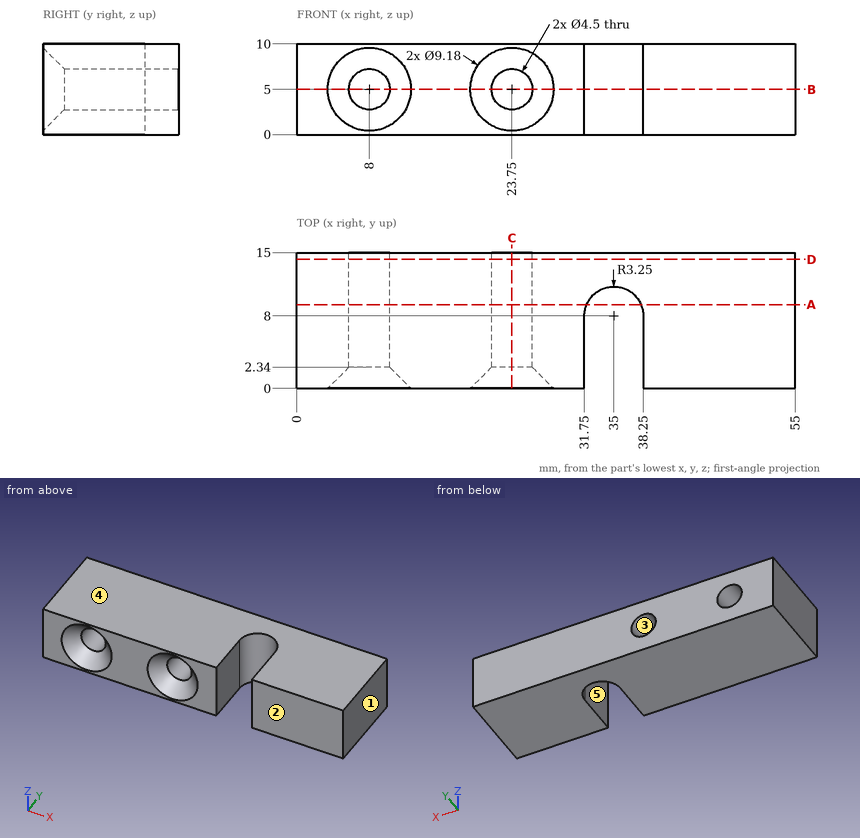
Geometry: see drawing. Coordinates: mm, zero at the bounding-box minimum. A direction names the side the tool comes from. Give positions to 0.01 mm unless a question says otherwise; leave off trailing zeros. Loops run counter-clockwise (first coordinate to the right, second up) from the corner with the lowest first, then second, coordinate; pieces in that order, holes last. Notation, with made-up numbers: (1, -37.75) -> (19, -37.75) arc R12 ccw to (19, -17.75) -> close; hole circle Ø2 at (-37.5, 75). An arc over 180 degrees is marked (long way). Answer as a JSON object with one key per item and string values. Group by question number.
Item 1: Cut plane D-D, the plane y = 14.25. Return the cut outline in (x, z), and give its area (3 significant figures).
Item 2: Cut plane B-B, the plane z = 5. Return the cut outline in (x, y).
Item 3: Pin query (flat end, axial travel): P1, Ø3.5, axis at x = 23.75, z = 5, coming from the +Y side. Return the tip coordinate at first contact, or that it passes through.
Item 4: Pull-direction query (X, two-part tool) for the marked faces 1, 2 and 3; classes: released by +X, released by -X, zero draft, split by the parting line, or undercut.
Item 5: Reachability of the marked faces 4 and 5 from +Z, -Z, +X, -X, +Y, -Y: full face, straight path, thin tool, end or side. Return the list, or none.
Item 6: Cut plane C-C, the plane x = 23.75. Return the cut outline in (y, z).
Item 7: Cut plane A-A, the plane y = 9.25. Return the cut outline in (x, z), and give its area (3 significant figures).
Item 8: Line query: probe 1 along X at (y, z) = (7, 5); probe 2 along X at (y, z) = (11.75, 5); probe 3 along X at (y, z) = (1.75, 2). Output: solid intervals per line, ascending.
Checks:
{
 "1": {"outline": "(0, 0) -> (55, 0) -> (55, 10) -> (0, 10) -> close; hole circle Ø4.5 at (8, 5); hole circle Ø4.5 at (23.75, 5)", "area": "518 mm²"},
 "2": {"outline": "(0, 0) -> (3.41, 0) -> (5.75, 2.34) -> (5.75, 15) -> (0, 15) -> close; (10.25, 2.34) -> (12.59, 0) -> (19.16, 0) -> (21.5, 2.34) -> (21.5, 15) -> (10.25, 15) -> close; (26, 2.34) -> (28.34, 0) -> (31.75, 0) -> (31.75, 8) arc R3.25 cw to (38.25, 8) -> (38.25, 0) -> (55, 0) -> (55, 15) -> (26, 15) -> close"},
 "3": {"P1": "passes through"},
 "4": {"face 1": "released by +X", "face 2": "zero draft", "face 3": "undercut"},
 "5": {"face 4": "+Z, +X, -X, +Y, -Y", "face 5": "+Z, -Z, -Y"},
 "6": {"outline": "(0, 0) -> (15, 0) -> (15, 2.75) -> (2.34, 2.75) -> (0, 0.41) -> close; (0, 9.59) -> (2.34, 7.25) -> (15, 7.25) -> (15, 10) -> (0, 10) -> close"},
 "7": {"outline": "(0, 0) -> (32, 0) -> (32, 10) -> (0, 10) -> close; (38, 0) -> (55, 0) -> (55, 10) -> (38, 10) -> close; hole circle Ø4.5 at (8, 5); hole circle Ø4.5 at (23.75, 5)", "area": "458 mm²"},
 "8": {"probe 1": "x = 0 to 5.75, 10.25 to 21.5, 26 to 31.75, 38.25 to 55", "probe 2": "x = 0 to 5.75, 10.25 to 21.5, 26 to 55", "probe 3": "x = 0 to 31.75, 38.25 to 55"}
}
